For this review, take the finished solid that the model builds, in its own axes (mm). Face numbers are marked on the shaded views. A direction names the side the tool comes from. Give positions to 0.01 mm unless a question says otherwise; leave off trailing zeros. Write each loop counter-clockwise with the first axis right and the second up, starting at its lowest first coordinate (ties: lowest second). Pieces come first, ordered by that corner, then holes. Notation, with made-up numbers: (53, -28) -> (79, -28) arc R14 ccw to (79, -1) -> close; hole circle Ø10 at (29, 2.5). An arc over 180 degrees is marked (long way). Write item = value, one per line.
```python
from build123d import *

# Parameters (mm, degrees)
F1_DEPTH = 63.5
F0_W     = 25.4
F0_H     = 19.05
F2_DEPTH = 25.4
F3_DEPTH = 7.9375
F5_R     = 6.35


with BuildPart() as f1:
    # F0 (on Front) → F1 (new body, symmetric)
    with BuildSketch(Plane.XZ):
        Polygon((22.225, 9.525), (-41.275, 9.525), (-41.275, -9.525), (41.275, -9.525), (41.275, 9.525), align=None)
    extrude(amount=F1_DEPTH, both=True)

    # F0 (on Front) → F2 (join, symmetric)
    with BuildSketch(Plane.XZ):
        with BuildLine():
            Line((22.225, 27.0002), (22.225, 9.525))
            Line((22.225, 9.525), (41.275, 9.525))
            Line((41.275, 9.525), (41.275, 27.0002))
            ThreePointArc((41.275, 27.0002), (45.9246798487, 38.2255201513), (57.15, 42.8752))
            Line((57.15, 42.8752), (60.325, 42.8752))
            Line((60.325, 42.8752), (60.325, 61.9252))
            Line((60.325, 61.9252), (57.15, 61.9252))
            ThreePointArc((57.15, 61.9252), (32.4542956671, 51.6959043329), (22.225, 27.0002))
        make_face()
        with Locations((73.025, 52.4002)):
            Rectangle(F0_W, F0_H)
    extrude(amount=F2_DEPTH, both=True)

    # F0 (on Front) → F3 (join, symmetric)
    with BuildSketch(Plane.XZ):
        with BuildLine():
            add(Edge.make_bspline(
                [(-41.275, 9.525), (-34.4362333417, 48.1805466115), (9.3027921394, 65.6224936247), (57.15, 61.9252)],
                knots=[0, 0, 0, 0, 111.5045361635, 111.5045361635, 111.5045361635, 111.5045361635], degree=3))
            Line((-41.275, 9.525), (22.225, 9.525))
            Line((22.225, 9.525), (22.225, 27.0002))
            ThreePointArc((22.225, 27.0002), (32.4542956671, 51.6959043329), (57.15, 61.9252))
        make_face()
    extrude(amount=F3_DEPTH, both=True)

    # F0 (on Front) → F4 (revolve)
    with BuildSketch(Plane.XZ):
        Polygon((85.725, 66.675), (85.725, 61.9252), (85.725, 42.8752), (85.725, 38.1), (111.125, 38.1), (111.125, 66.675), align=None)
    revolve(axis=Axis((85.725, 0, 52.3875), (0, 0, 1)))

    # F5
    f5_edges = [f1.edges().sort_by_distance(p)[0] for p in [
        (-41.275, -63.5, 0),
        (41.275, -63.5, 0),
        (41.275, 63.5, 0),
        (-41.275, 63.5, 0),
    ]]
    fillet(f5_edges, radius=F5_R)


with BuildPart() as f6_1:
    # F6: copy of F1
    add(f1.part.moved(Location((127, 127, 127))))


solid = f6_1.part
```
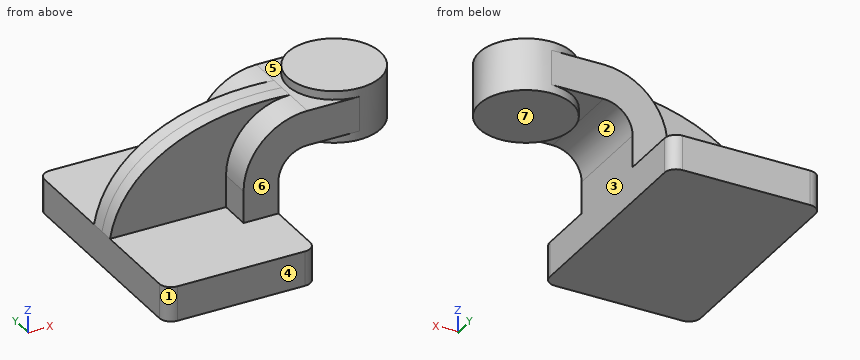
(1) Take a section at B-B (y = 139). Write out the cut boundary in (x, z) (3 decimals), plus the area to 3 significant figures.
Answers below:
outline = (85.725, 117.475) -> (168.275, 117.475) -> (168.275, 154) arc R15.875 cw to (184.15, 169.875) -> (190.338, 169.875) -> (190.338, 165.1) -> (235.112, 165.1) -> (235.112, 193.675) -> (190.338, 193.675) -> (190.338, 188.925) -> (184.15, 188.925) arc R34.925 ccw to (149.225, 154) -> (149.225, 136.525) -> (85.725, 136.525) -> close
area = 4,060 mm^2
(2) The part is to be moulded in two halves that separate along X. For the marked faces 1, 2, 3 and 4, say which applies: released by +X, released by -X, zero draft, split by the parting line, or undercut.
Answers below:
face_1 = released by -X
face_2 = undercut
face_3 = released by +X
face_4 = zero draft
(3) Take a section at C-C (y = 75). Write out the cut boundary in (x, z) (3 decimals).
Answers below:
outline = (85.725, 117.475) -> (168.275, 117.475) -> (168.275, 136.525) -> (85.725, 136.525) -> close
(4) To check wall thickness, follow probe 1 along Y at (x, z) = (140, 179.5); probe 2 along Z at (x, y) = (186, 118.5); probe 3 along Z at (x, y) = (108, 180) (3 decimals). State the ranges of each line that lie inside material, in increasing order.
Answers below:
probe_1 = 119.06 to 134.94
probe_2 = 169.88 to 188.93
probe_3 = 117.475 to 136.525
(5) For pin 1 (14.5 mm diameter, centred on x = 194.5, y = 130.5, fed in from -Z); pin 2 (2 mm diameter, centred on x = 133, z = 164, fed in from -Y); pin 3 (3 mm diameter, centred on x = 132, y = 129, fed in from +Z), all flat-tipped, find the tip position at first contact; note any pin that passes through.
Answers below:
pin_1 = 165.1
pin_2 = 119.06
pin_3 = 184.08
(6) Tool access review of the marked faces 5, 6 and 7: name each direction out of +Z, -Z, +X, -X, +Y, -Y from which nothing blocks a thin tool from reaching the whole face with its end or side.
Answers below:
face_5 = +Z
face_6 = +Z, +X, -X, -Y
face_7 = -Z, +X, +Y, -Y
(7) Take a section at A-A (x = 192). Write out the cut boundary in (y, z) (1 decimal), plus the area to 3 significant figures.
Answers below:
outline = (101.6, 169.9) -> (112.3, 169.9) -> (112.3, 165.1) -> (141.7, 165.1) -> (141.7, 169.9) -> (152.4, 169.9) -> (152.4, 188.9) -> (141.7, 188.9) -> (141.7, 193.7) -> (112.3, 193.7) -> (112.3, 188.9) -> (101.6, 188.9) -> close
area = 1,250 mm^2
